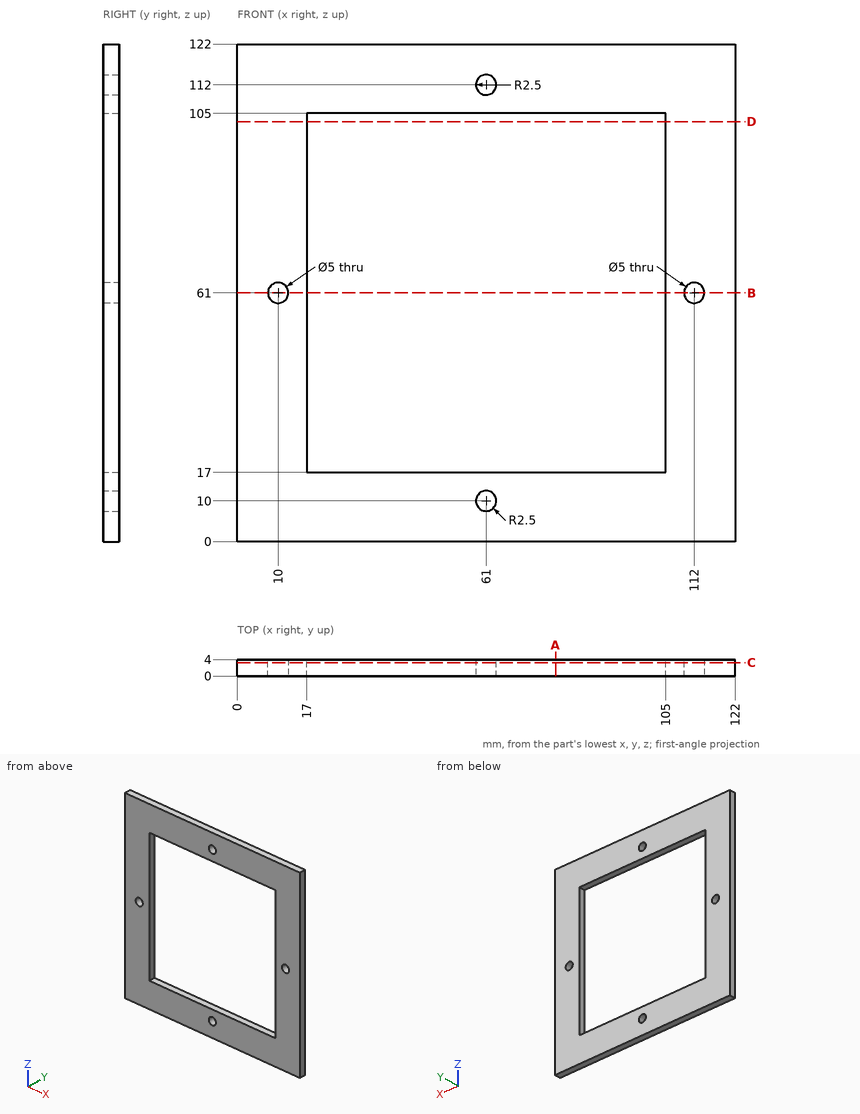
Study the drawing (mm; zero at the part's minimum x, y, z) and answer. Give positions to 0.01 mm unless a question says otherwise; leave off trailing zeros. Loops run counter-clockwise (first coordinate to the right, second up) from the corner with the lowest first, then second, coordinate; pieces in that order, holes last. Notation, with made-up numbers: (22.25, -37.5) - (68.25, -37.5) arc R24 ccw to (68.25, -12.5) - close; hole circle Ø7 at (-24.75, -32.75). An arc over 180 degrees is marked (long way). One line per question, with ' | ' between items.
(1) The part is cut by section D-D (z = 103). Write down the section's boundary in (x, y), then the cut area to 3 significant figures.
Recorded:
outline: (0, 0) - (17, 0) - (17, 4) - (0, 4) - close; (105, 0) - (122, 0) - (122, 4) - (105, 4) - close | area: 136 mm²
(2) The part is cut by section A-A (x = 78). Write down the section's boundary in (y, z), then the cut area to 3 significant figures.
Recorded:
outline: (0, 0) - (4, 0) - (4, 17) - (0, 17) - close; (0, 105) - (4, 105) - (4, 122) - (0, 122) - close | area: 136 mm²
(3) The part is cut by section C-C (y = 3.3). Write down the section's boundary in (x, z), then the cut area to 3 significant figures.
Recorded:
outline: (0, 0) - (122, 0) - (122, 122) - (0, 122) - close; hole circle Ø5 at (10, 61); hole (17, 17) - (105, 17) - (105, 105) - (17, 105) - close; hole circle Ø5 at (61, 10); hole circle Ø5 at (61, 112); hole circle Ø5 at (112, 61) | area: 7,060 mm²
(4) Straight lines are drawn through the part: probe 1 along X at (y, z) = (1.6, 61); probe 2 along X at (y, z) = (2.9, 21). For each, find the intervals that lie inside material, in ascending order.
Recorded:
probe 1: x = 0 to 7.5, 12.5 to 17, 105 to 109.5, 114.5 to 122 | probe 2: x = 0 to 17, 105 to 122
(5) This flat-tipped pin is pushed along its axis until it touches: pin 1 Ø1.2 at (y, z) = (1.5, 75) entering from -X. Where does it stop, or does it pass through?
Recorded:
pin 1: stops at x = 0
(6) The part is cut by section B-B (z = 61). Write down the section's boundary in (x, y), then the cut area to 3 significant figures.
Recorded:
outline: (0, 0) - (7.5, 0) - (7.5, 4) - (0, 4) - close; (12.5, 0) - (17, 0) - (17, 4) - (12.5, 4) - close; (105, 0) - (109.5, 0) - (109.5, 4) - (105, 4) - close; (114.5, 0) - (122, 0) - (122, 4) - (114.5, 4) - close | area: 96.0 mm²
